from build123d import *

# Parameters (mm, degrees)
CROQUIS1_R              = 2
SALIENTE_EXTRUIR1_DEPTH = 5
CROQUIS3_R              = 2
SALIENTE_EXTRUIR2_DEPTH = 5
CROQUIS5_R              = 2
SALIENTE_EXTRUIR3_DEPTH = 5
CROQUIS6_R              = 2
SALIENTE_EXTRUIR4_DEPTH = 5


with BuildPart() as part:
    # Croquis1 → Saliente-Extruir1 (new body)
    with BuildSketch(Plane.XY):
        with BuildLine():
            Line((-52.02, -10), (-26.01, -10))
            Line((-26.01, -10), (-26.01, 10))
            Line((-26.01, 10), (-52.02, 10))
            ThreePointArc((-52.02, 10), (-62.02, 0), (-52.02, -10))
        make_face()
        with Locations((-52.02, 0)):
            Circle(CROQUIS1_R, mode=Mode.SUBTRACT)
        with BuildLine():
            Line((-26.01, 10), (-26.01, -10))
            Line((-26.01, -10), (0, -10))
            ThreePointArc((0, -10), (10, 0), (0, 10))
            Line((0, 10), (-26.01, 10))
        make_face()
        Circle(CROQUIS1_R, mode=Mode.SUBTRACT)
    extrude(amount=SALIENTE_EXTRUIR1_DEPTH)



with BuildPart() as body_2:
    # Croquis3 → Saliente-Extruir2 (new body)
    with BuildSketch(Plane.XY.offset(13)):
        with BuildLine():
            Line((-52.02, 10), (0, 10))
            ThreePointArc((0, 10), (10, 0), (0, -10))
            Line((0, -10), (-52.02, -10))
            ThreePointArc((-52.02, -10), (-62.02, 0), (-52.02, 10))
        make_face()
        with Locations((-52.02, 0)):
            Circle(CROQUIS3_R, mode=Mode.SUBTRACT)
        Circle(CROQUIS3_R, mode=Mode.SUBTRACT)
    extrude(amount=SALIENTE_EXTRUIR2_DEPTH)


with BuildPart() as part_1:
    add(part.part)

    add(body_2.part)  # Saliente-Extruir3 merges body 2
    # Croquis5 → Saliente-Extruir3 (add)
    with BuildSketch(Plane(origin=(-17.01, 10, 0), x_dir=(0, 0, -1), z_dir=(1, 0, 0))):
        with BuildLine():
            Line((-35.01, -20), (17.01, -20))
            ThreePointArc((17.01, -20), (27.01, -10), (17.01, 0))
            Line((17.01, 0), (-35.01, 0))
            ThreePointArc((-35.01, 0), (-45.01, -10), (-35.01, -20))
        make_face()
        with Locations((17.01, -10)):
            Circle(CROQUIS5_R, mode=Mode.SUBTRACT)
        with Locations((-35.01, -10)):
            Circle(CROQUIS5_R, mode=Mode.SUBTRACT)
    extrude(amount=-SALIENTE_EXTRUIR3_DEPTH)

    # Croquis6 → Saliente-Extruir4 (add)
    with BuildSketch(Plane(origin=(-35.01, 10, 0), x_dir=(0, 0, -1), z_dir=(1, 0, 0))):
        with BuildLine():
            Line((17.01, 0), (-9, 0))
            Line((-9, 0), (-9, -20))
            Line((-9, -20), (17.01, -20))
            ThreePointArc((17.01, -20), (27.01, -10), (17.01, 0))
        make_face()
        with Locations((17.01, -10)):
            Circle(CROQUIS6_R, mode=Mode.SUBTRACT)
        with BuildLine():
            Line((-9, -20), (-9, 0))
            Line((-9, 0), (-35.01, 0))
            ThreePointArc((-35.01, 0), (-45.01, -10), (-35.01, -20))
            Line((-35.01, -20), (-9, -20))
        make_face()
        with Locations((-35.01, -10)):
            Circle(CROQUIS6_R, mode=Mode.SUBTRACT)
    extrude(amount=SALIENTE_EXTRUIR4_DEPTH)


solid = part_1.part
Geometry check sheet. Reference: the model listing, model coordinates, mm. A direction names the side the tool comes from. Round coordinates to 2 decimals unless told otherwise and drop trailing zeros. Loops run counter-clockwise (first coordinate to the right, second up) from the corner with the lowest first, then second, coordinate; pieces in that order, holes last. Notation, with made-up numbers: (-33.5, 49.5) -> (17.5, 49.5) arc R12 cw to (17.5, 60.5) -> close; hole circle Ø2 at (49, 78). An arc over 180 degrees is marked (long way). Answer as a JSON object with one key per item and string values. Group by question number.
Item 1: Thickness scan on line 1 along X through (y, z) = (2.75, -19); line 2 along Z through (x, y) = (-40.5, -2.5); line 3 along Y through (x, z) = (-20, -17). Record the ranges inside material, lowest first.
Item 2: Depth check by flat-ended pin: pin 1 Ø5 at (y, z) = (0, -17.01) entering from -X; pin 2 Ø6.5 at (x, y) = (0, 0) entering from -Z; pin 3 Ø5 at (x, y) = (0, 0) entering from +Z; pin 4 Ø2.5 at (y, z) = (0, -17.01) entering from +X. Enter the tip coordinate at first touch or a pass-through.
Item 3: Cross-section at C-C, the plane z = 40. Record the cut outline in (x, y).
Item 4: Cross-section at B-B, the plane y = 0. Count the separate pieces of the cut face and the enclosed holes in it, plus the area to 3 significant figures.
Item 5: Cross-section at A-A, the plane x = -23. Record the cut outline in (y, z), plus the area to 3 significant figures.
Item 6: Set-up check for faces 4 (the face through (-26, 0, 13)), 5 (the face through (-26, 0, 18)), 6 (the face through (-4, 0, 5)), 7 (the face through (-35.01, 0, -13)), 8 (the face through (-26, 0, 0)): record each of +Z, -Z, +X, -X, +Y, -Y from which the full face is reachable in a straight line by a thin tool's end or side.
Item 7: Release check for a two-part mould opening along X. For faces 1 (the face through (-26, 0, 5)), 2 (the face through (-17.01, 0, 32)), 3 (the face through (-48, 0, 13)) record: pulls with the +X half, pulls with the -X half, needs draft (parallel to the pull), parting line crosses it, or undercut.
Determined:
{
 "1": {"line 1": "x = -35.01 to -30.01, -22.01 to -17.01", "line 2": "z = 0 to 5, 13 to 18", "line 3": "y = -10 to -2, 2 to 10"},
 "2": {"pin 1": "stops at x = -35.01", "pin 2": "stops at z = 0", "pin 3": "stops at z = 18", "pin 4": "passes through"},
 "3": {"outline": "(-35.01, -8.67) -> (-30.01, -8.67) -> (-30.01, 8.67) -> (-35.01, 8.67) -> close; (-22.01, -8.67) -> (-17.01, -8.67) -> (-17.01, 8.67) -> (-22.01, 8.67) -> close"},
 "4": {"separate pieces": "9", "enclosed holes": "1", "area": "1,180 mm²"},
 "5": {"outline": "(-10, 0) -> (10, 0) -> (10, 5) -> (-10, 5) -> close; (-10, 13) -> (10, 13) -> (10, 18) -> (-10, 18) -> close", "area": "200 mm²"},
 "6": {"face 4": "+Y, -Y", "face 5": "+Z, +Y, -Y", "face 6": "+X, +Y, -Y", "face 7": "-Z, -X, +Y, -Y", "face 8": "-Z, +Y, -Y"},
 "7": {"face 1": "undercut", "face 2": "pulls with the +X half", "face 3": "needs draft"}
}
